Read the model definition and answer for the solid it produces. Units are mm, in the model's axes. Coordinates: 2 decimals unless noted, no trailing zeros. Loops run counter-clockwise (first coordinate to the right, second up) from the corner with the lowest first, then second, coordinate; pieces in that order, holes last.
from build123d import *

# Parameters (mm, degrees)
SKETCH1_R           = 1.5
SKETCH1_R_2         = 1
SKETCH1_R_3         = 7.502494881
BOSS_EXTRUDE2_DEPTH = 1.5


with BuildPart() as part:
    # Sketch1 → Boss-Extrude2 (new body)
    with BuildSketch(Plane.XY):
        Polygon((89.453108516, 4.337043032), (-1.643229796, 4.337043032), (-3.057443358, 2.92282947), (-3.057443358, -88.173508842), (-1.643229796, -89.587722405), (89.453108516, -89.587722405), (90.867322078, -88.173508842), (90.867322078, -53.341657496), (92.281535641, -51.927443934), (101.643338186, -51.927443934), (103.057551748, -50.513230371), (103.057551748, -8.692923399), (101.643338186, -7.278709837), (90.867322078, -7.278709837), (90.867322078, 2.92282947), align=None)
        with Locations((7.002900718, -1.018478259)):
            Circle(SKETCH1_R, mode=Mode.SUBTRACT)
        with Locations((27.371818874, -1.018478259)):
            Circle(SKETCH1_R, mode=Mode.SUBTRACT)
        with Locations((34.50904124, -0.868109843)):
            Circle(SKETCH1_R_2, mode=Mode.SUBTRACT)
        with Locations((57.413525643, -0.868109843)):
            Circle(SKETCH1_R_2, mode=Mode.SUBTRACT)
        with Locations((87.07937983, 0.003106997)):
            Circle(SKETCH1_R_2, mode=Mode.SUBTRACT)
        with Locations((68.250695172, -17.55885203)):
            Circle(SKETCH1_R_3, mode=Mode.SUBTRACT)
        with Locations((7.002900718, -44.317247133)):
            Circle(SKETCH1_R, mode=Mode.SUBTRACT)
        with Locations((27.371818874, -44.317247133)):
            Circle(SKETCH1_R, mode=Mode.SUBTRACT)
        with Locations((0, -86.555222321)):
            Circle(SKETCH1_R_2, mode=Mode.SUBTRACT)
        with Locations((87.07937983, -86.555222321)):
            Circle(SKETCH1_R_2, mode=Mode.SUBTRACT)
        Circle(SKETCH1_R_2, mode=Mode.SUBTRACT)
    extrude(amount=BOSS_EXTRUDE2_DEPTH)


solid = part.part
Q1. A cutting plane is placed at A-A (x = 68.5). Give the vertices of the cut face in (y, z), then the cut area to 3 significant figures.
Findings below:
outline: (-89.59, 0) - (-25.06, 0) - (-25.06, 1.5) - (-89.59, 1.5) - close; (-10.06, 0) - (4.34, 0) - (4.34, 1.5) - (-10.06, 1.5) - close
area: 118 mm2
Q2. Straight lines are drawn through the part: probe 1 along X at (y, z) = (-17.5, 1.3); probe 2 along X at (y, z) = (-64, 1.4); probe 3 along X at (y, z) = (-45, 0.65). For each, find the intervals that lie inside material, in ascending order.
Findings below:
probe 1: x = -3.06 to 60.75, 75.75 to 103.06
probe 2: x = -3.06 to 90.87
probe 3: x = -3.06 to 5.67, 8.34 to 26.04, 28.71 to 103.06
Q3. A cutting plane is placed at B-B (z = 1.25). Count the separate pieces of the cut face and the enclosed holes in it, then the cut area to 3 significant figures.
Findings below:
separate pieces: 1
enclosed holes: 11
area: 9,140 mm2
Q4. Flat-ended cylindrical pins translate along their axes: pin 1 Ø1.6 at (x, y) = (87.08, 0) entering from -Z; pin 2 Ø0.8 at (y, z) = (-64, 0.5) entering from +X. Find the tip coordinate at first contact, or state that the pin passes through.
Findings below:
pin 1: passes through
pin 2: stops at x = 90.87
Q5. A cutting plane is placed at C-C (y = -61.5). Give the vertices of the cut face in (x, z), then the cut area to 3 significant figures.
Findings below:
outline: (-3.06, 0) - (90.87, 0) - (90.87, 1.5) - (-3.06, 1.5) - close
area: 141 mm2
Q6. Determine the mould class of faces 1 (the face through (49, -42, 0)), 2 (the face through (25.873, -0.953, 0.74)) for opening direction Y: +Y half, -Y half, draft (parallel to the pull), parting line (faces both ways), or undercut.
Findings below:
face 1: draft
face 2: undercut
